from build123d import *

# Parameters (mm, degrees)
BOSS_EXTRU_1_DEPTH      = 12
ESQUISSE2_R             = 9.1
ENL_V_MAT_EXTRU_3_DEPTH = 8
ENL_V_MAT_EXTRU_4_DEPTH = 6
ENL_V_MAT_EXTRU_5_DEPTH = 0.8
BOSS_EXTRU_2_DEPTH      = 12
ESQUISSE6_R             = 1.9
ENL_V_MAT_EXTRU_6_DEPTH = 10
CONG_1_R                = 5
CONG_2_R                = 2


with BuildPart() as part:
    # Esquisse1 → Boss.-Extru.1 (new body)
    with BuildSketch(Plane.XY):
        with BuildLine():
            Line((10.392304845, 6), (20, 6))
            Line((20, 6), (20, -6))
            Line((20, -6), (10.392304845, -6))
            ThreePointArc((10.392304845, -6), (-12, 0), (10.392304845, 6))
        make_face()
    extrude(amount=BOSS_EXTRU_1_DEPTH)

    # Esquisse2 → Enlèv. mat.-Extru.3 (cut)
    with BuildSketch(Plane.XY.offset(12)):
        Circle(ESQUISSE2_R)
    extrude(amount=-ENL_V_MAT_EXTRU_3_DEPTH, mode=Mode.SUBTRACT)

    # Esquisse3 → Enlèv. mat.-Extru.4 (cut)
    with BuildSketch(Plane.XY.offset(12)):
        with BuildLine():
            Line((9.644169223, 3), (17, 3))
            Line((17, 3), (17, -3))
            Line((17, -3), (9.644169223, -3))
            ThreePointArc((9.644169223, -3), (10.1, 0), (9.644169223, 3))
        make_face()
    extrude(amount=-ENL_V_MAT_EXTRU_4_DEPTH, mode=Mode.SUBTRACT)

    # Esquisse4 → Enlèv. mat.-Extru.5 (cut)
    with BuildSketch(Plane.XY.offset(12)):
        with BuildLine():
            Line((17, -3), (17, 3))
            Line((17, 3), (9.644169223, 3))
            ThreePointArc((9.644169223, 3), (-10.1, 0), (9.644169223, -3))
            Line((9.644169223, -3), (17, -3))
        make_face()
    extrude(amount=-ENL_V_MAT_EXTRU_5_DEPTH, mode=Mode.SUBTRACT)

    # Esquisse5 → Boss.-Extru.2 (add)
    with BuildSketch(Plane.XY.offset(12)):
        with BuildLine():
            Line((20, 6), (20, -6))
            ThreePointArc((20, -6), (26, 0), (20, 6))
        make_face()
        with BuildLine():
            Line((-10.857142857, 5.11101252), (-10.857142857, -5.11101252))
            ThreePointArc((-10.857142857, -5.11101252), (-20, 0), (-10.857142857, 5.11101252))
        make_face()
    extrude(amount=-BOSS_EXTRU_2_DEPTH)

    # Esquisse6 → Enlèv. mat.-Extru.6 (cut)
    with BuildSketch(Plane.XY.offset(12)):
        with Locations((-14, 0)):
            Circle(ESQUISSE6_R)
        with Locations((20, 0)):
            Circle(ESQUISSE6_R)
    extrude(amount=-ENL_V_MAT_EXTRU_6_DEPTH, mode=Mode.SUBTRACT)

    # Congé1
    cong_1_edges = [part.edges().sort_by_distance(p)[0] for p in [
        (9.644169223, 3, 11.6),
        (9.644169223, -3, 11.6),
    ]]
    fillet(cong_1_edges, radius=CONG_1_R)

    # Congé2
    cong_2_edges = [part.edges().sort_by_distance(p)[0] for p in [
        (17, 3, 9),
        (17, -3, 9),
        (-10.857142857, -5.11101252, 6),
        (-10.857142857, 5.11101252, 6),
        (10.392304845, 6, 6),
        (10.392304845, -6, 6),
    ]]
    fillet(cong_2_edges, radius=CONG_2_R)


solid = part.part
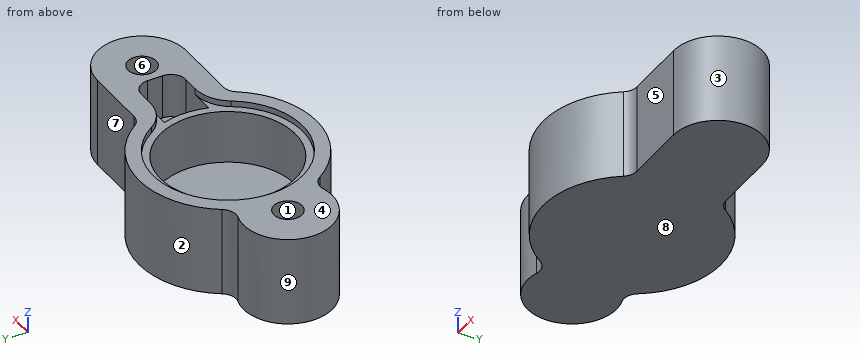
Could you check a few things on this model? Use its own coordinates, in mm. Face numbers are marked on the shaded views. A direction names the side the tool comes from. Give positions to 0.01 mm unless a question says otherwise; leave off trailing zeros. Order: outer loops, then holes, each group sorted by start corner. A loop starts at its lowest first (then second) coordinate and runs counter-clockwise, first axis right, second up.
Item 1: I'm going to push flat-ended pins straight in: pin 1 (1.5 mm diameter, centred on x = -6.5, y = 7.5, fed in from +Z); pin 2 (4.5 mm diameter, centred on x = 16.5, z = 6, fed in from -Y); pin 3 (1.6 mm diameter, centred on x = 12.5, z = 10.5, fed in from +Y); pin 4 (6 mm diameter, centred on x = 12, z = 2, fed in from +Y). Where does each tip first touch, or does it pass through?
Item 2: If we mould it in two halves opening along X, with no side actions, what happens to the marked faces 1, 2, 3 and 4? For each: pulls with the +X half, pulls with the -X half, needs draft (parallel to the pull), parting line crosses it, or undercut.
Item 3: I need wall thicknesses on line 1 (Y direction, x = 20, z = 5.75); line 2 (Y direction, x = 15, z = 6.25); line 3 (Z direction, x = 15, y = 2.25). Which ranges of each line are inside material? Lowest first, please.
Item 4: For the marked faces 5, 6, 7, 8 and 9, which set-ups out of +Z, -Z, +X, -X, +Y, -Y let a thin tool reach every point of the face, with its end or its side?
Item 5: If we section it at D-D, the plane z = 5.5: Count the separate pieces of the cut face and the enclosed holes in it, plus the area to 3 significant figures.
Item 6: If we section it at B-B, the plane y = 0: Write out the boundary of the cut face in (x, z).
Item 7: If we section it at A-A, the plane x = -14: Write out the boundary of the cut face in (y, z), plus the area to 3 significant figures.
Item 8: If we section it at C-C, the plane x = 0: Write out the boundary of the cut face in (y, z).
Values:
1. pin 1: stops at z = 12
1. pin 2: stops at y = -6
1. pin 3: stops at y = 6
1. pin 4: stops at y = 7.94
2. face 1: undercut
2. face 2: parting line crosses it
2. face 3: pulls with the +X half
2. face 4: needs draft
3. line 1: y = -6 to -1.9, 1.9 to 6
3. line 2: y = -6 to -3, 3 to 6
3. line 3: z = 0 to 6
4. face 5: +Z, -Z, +X, -Y
4. face 6: +Z
4. face 7: +Z, -Z, +X, +Y
4. face 8: -Z, +X, -X, +Y, -Y
4. face 9: +Z, -Z
5. separate pieces: 1
5. enclosed holes: 3
5. area: 414 mm2
6. outline: (-20, 0) - (26, 0) - (26, 12) - (21.9, 12) - (21.9, 2) - (18.1, 2) - (18.1, 12) - (17, 12) - (17, 6) - (10.1, 6) - (10.1, 11.2) - (9.1, 11.2) - (9.1, 4) - (-9.1, 4) - (-9.1, 11.2) - (-10.1, 11.2) - (-10.1, 12) - (-12.1, 12) - (-12.1, 2) - (-15.9, 2) - (-15.9, 12) - (-20, 12) - close
7. outline: (-6, 0) - (6, 0) - (6, 12) - (1.9, 12) - (1.9, 2) - (-1.9, 2) - (-1.9, 12) - (-6, 12) - close
7. area: 106 mm2
8. outline: (-12, 0) - (12, 0) - (12, 12) - (10.1, 12) - (10.1, 11.2) - (9.1, 11.2) - (9.1, 4) - (-9.1, 4) - (-9.1, 11.2) - (-10.1, 11.2) - (-10.1, 12) - (-12, 12) - close
